Geometry: see drawing. Coordinates: mm, zero at the bounding-box minimum. A direction names the side the tool comes from. Coordinates: 2 decimals unless noted, no trailing zeros. Loops run counter-clockwise (first coordinate to the right, second up) from the corner with the lowest first, then second, coordinate; pieces in that order, holes last. Notation, with made-up numbers: (2, 69.5) - (19, 69.5) arc R17 ccw to (19, 86.5) - close; hole circle Ø10 at (-1, 29). An arc over 180 degrees is marked (long way). Answer in a Markdown table with one row per item.
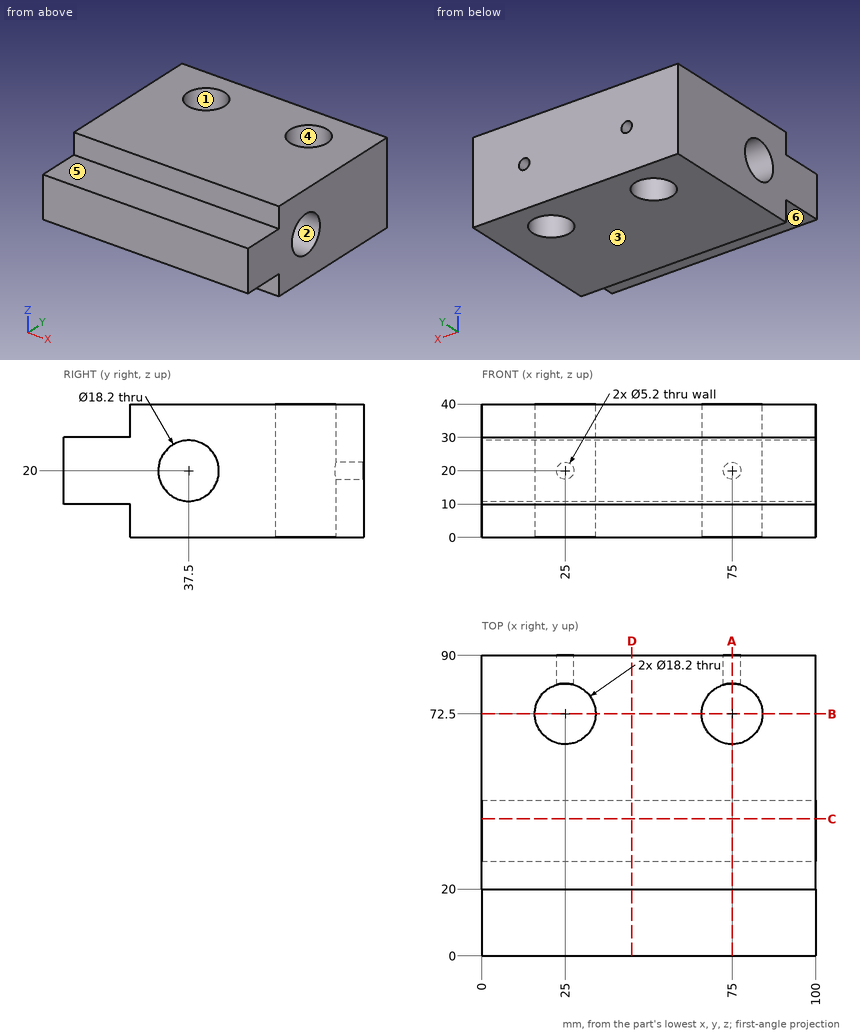
(1) Cut plane C-C on y = 41. Output: boundary loops of the cut face in (x, z), then the cut area to 3 significant figures.
Verdict:
| item | result |
|---|---|
| outline | (0, 0) - (100, 0) - (100, 11.6) - (0, 11.6) - close; (0, 28.4) - (100, 28.4) - (100, 40) - (0, 40) - close |
| area | 2,320 mm² |
(2) First-contact query: pin 1 Ø3 at (x, z) = (75, 20) entering from +Y; pin 2 Ø8 at (x, z) = (28, 37) entering from -Y; pin 3 Ø16.5 at (y, z) = (37.5, 20) entering from +X; pin 4 Ø4 at (x, z) = (25, 20) entering from +Y. Flat tips, straight axial feed; report the tip coordinate or a pass-through.
Verdict:
| item | result |
|---|---|
| pin 1 | stops at y = 63.52 |
| pin 2 | stops at y = 20 |
| pin 3 | passes through |
| pin 4 | stops at y = 63.62 |
(3) Cut plane D-D on x = 45. Output: boundary loops of the cut face in (y, z), then the cut area to 3 significant figures.
Verdict:
| item | result |
|---|---|
| outline | (0, 10) - (20, 10) - (20, 0) - (90, 0) - (90, 40) - (20, 40) - (20, 30) - (0, 30) - close; hole circle Ø18.2 at (37.5, 20) |
| area | 2,940 mm² |
(4) Cut plane A-A on x = 75. Output: boundary loops of the cut face in (y, z), then the cut area to 3 significant figures.
Verdict:
| item | result |
|---|---|
| outline | (0, 10) - (20, 10) - (20, 0) - (63.4, 0) - (63.4, 40) - (20, 40) - (20, 30) - (0, 30) - close; (81.6, 0) - (90, 0) - (90, 17.4) - (81.6, 17.4) - close; (81.6, 22.6) - (90, 22.6) - (90, 40) - (81.6, 40) - close; hole circle Ø18.2 at (37.5, 20) |
| area | 2,170 mm² |
(5) Pull-direction query (Z, two-part tool) for the marked faces 1, 2 and 3; classes: pulls with the +Z half, pulls with the -Z half, needs draft (parallel to the pull), parting line crosses it, or undercut.
Verdict:
| item | result |
|---|---|
| face 1 | needs draft |
| face 2 | undercut |
| face 3 | pulls with the -Z half |
(6) Ray query, probe 1 along X at (y, z) = (72.5, 26.5); probe 2 along Y at (x, z) = (65, 20); probe 3 along X at (y, z) = (71, 8). Return the intervals inside material, ascending.
Verdict:
| item | result |
|---|---|
| probe 1 | x = 0 to 15.9, 34.1 to 65.9, 84.1 to 100 |
| probe 2 | y = 0 to 28.4, 46.6 to 90 |
| probe 3 | x = 0 to 16.02, 33.98 to 66.02, 83.98 to 100 |
(7) Access query for the marked faces 4, 5 and 6. Directions: +Z, -Z, +X, -X, +Y, -Y. A direction counts if a zero-diameter tool reaches every point of the face in a straight line with its end or side. Return the directions, or none.
Verdict:
| item | result |
|---|---|
| face 4 | +Z, -Z |
| face 5 | +Z, +X, -X, -Y |
| face 6 | -Z, +X, -X, -Y |
(8) Cut plane B-B on y = 72.5. Output: boundary loops of the cut face in (x, z), then the cut area to 3 significant figures.
Verdict:
| item | result |
|---|---|
| outline | (0, 0) - (15.9, 0) - (15.9, 40) - (0, 40) - close; (34.1, 0) - (65.9, 0) - (65.9, 40) - (34.1, 40) - close; (84.1, 0) - (100, 0) - (100, 40) - (84.1, 40) - close |
| area | 2,540 mm² |
